Work out the finished part from the listing and answer in its coordinate system (mm). Coordinates: 2 decimals unless noted, no trailing zeros. Order: outer loops, then holes, each group sorted by start corner. A loop starts at its lowest first (then second) coordinate and runs counter-clockwise, first axis right, second up. Notation, with made-up numbers: M 53.25,18.25 L 91.25,18.25 A32 ccw 91.25,48.25 Z; hole C 58,67.25 d10. An arc over 180 degrees is marked long. Answer in a Markdown table with one row per item. Add a question column.
Item 1: The part is cut by section A-A (y = 0.1). Write down the section's boundary in (x, z), then the cut area to 3 significant figures.
Item 2: The part is cut by section D-D (z = 4). Write down the section's boundary in (x, y).
Item 3: The part is cut by section B-B (x = -4.5). Write down the section's boundary in (y, z), then the cut area to 3 significant figures.
Item 4: Consider line 1 (X direction, y = 0.15, z = -2.5); line 2 (X direction, y = 0.25, z = 2.5); line 3 (Z direction, x = -3, y = 0.1). Determine where each line is inside the solid, lowest interval first. Write a range as from..to.
Item 5: The part is cut by section C-C (z = -3). Write down the section's boundary in (x, y).
from build123d import *

# Parameters (mm, degrees)
F1_DEPTH = 0.508


with BuildPart() as f1:
    # F0 (on Front) → F1 (new body)
    with BuildSketch(Plane.XZ):
        Polygon((22.398183, 21.82091), (-24.014546, 21.82091), (0, -20.666365), align=None)
        Polygon((9.164905, 4.574282), (0, -14.431817), (-10.435999, 4.657122), (-6.927273, 6.119091), (0, -10.506364), (6.234545, 6.119091), align=None, mode=Mode.SUBTRACT)
    extrude(amount=-F1_DEPTH)


solid = f1.part
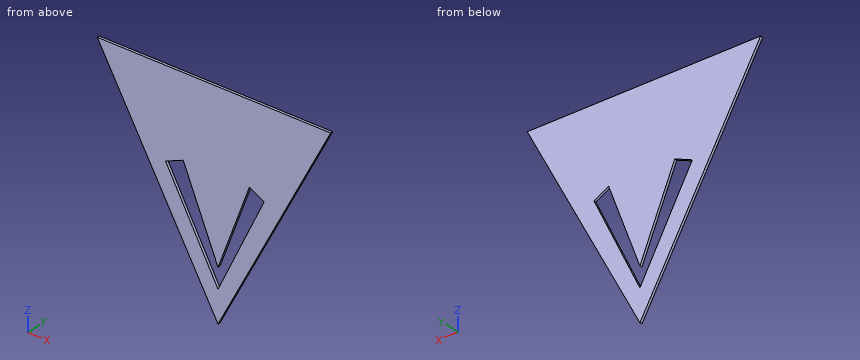
Reply:
| question | item | result |
|---|---|---|
| 1 | outline | M -24.01,21.82 L 0,-20.67 L 22.4,21.82 Z; hole M -10.44,4.66 L 0,-14.43 L 9.16,4.57 L 6.23,6.12 L 0,-10.51 L -6.93,6.12 Z |
| 1 | area | 884 mm2 |
| 2 | outline | M -13.94,0 L -10.08,0 L -10.08,0.51 L -13.94,0.51 Z; M -6.04,0 L 5.44,0 L 5.44,0.51 L -6.04,0.51 Z; M 8.89,0 L 13,0 L 13,0.51 L 8.89,0.51 Z |
| 3 | outline | M 0,-12.7 L 0.51,-12.7 L 0.51,-6.2 L 0,-6.2 Z; M 0,0.29 L 0.51,0.29 L 0.51,21.82 L 0,21.82 Z |
| 3 | area | 14.2 mm2 |
| 4 | line 1 | x = -10.27..-6.52, -3.34..3, 5.75..9.58 |
| 4 | line 2 | x = -13.09..-9.26, -5.42..4.88, 8.16..12.21 |
| 4 | line 3 | z = -15.36..-8.94, -3.31..21.82 |
| 5 | outline | M -9.99,0 L -6.25,0 L -6.25,0.51 L -9.99,0.51 Z; M -3.13,0 L 2.81,0 L 2.81,0.51 L -3.13,0.51 Z; M 5.51,0 L 9.31,0 L 9.31,0.51 L 5.51,0.51 Z |
